Source: CAD feature listing. Evaluate the final solid. Frame: model axes, mm. Face numbers are marked on the shaded views. A direction names the side the tool comes from. Give positions to 0.01 mm unless a question says otherwise; leave off trailing zeros. Order: outer loops, then holes, each group sorted by start corner. A loop starts at its lowest first (then second) coordinate and runs counter-clockwise, first axis right, second up.
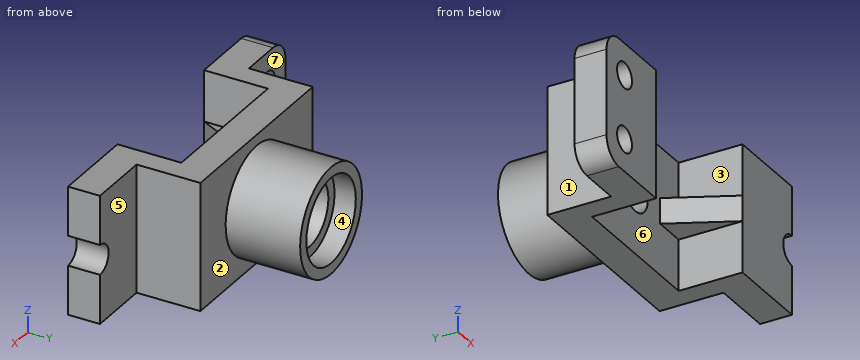
```python
from build123d import *

# Parameters (mm, degrees)
BOSS_EXTRUDE1_DEPTH = 30
BOSS_EXTRUDE2_DEPTH = 6
SKETCH3_R           = 6
CUT_EXTRUDE1_DEPTH  = 87.168439698
FILLET1_R           = 10
SKETCH4_R           = 7
CUT_EXTRUDE2_DEPTH  = 22
SKETCH5_R           = 25
BOSS_EXTRUDE3_DEPTH = 35
SKETCH6_R           = 20
CUT_EXTRUDE3_DEPTH  = 10
SKETCH7_R           = 15
SKETCH8_R           = 10


with BuildPart() as part:
    # Sketch1 → Boss-Extrude1 (new, symmetric)
    with BuildSketch(Plane.XY):
        Polygon((-75, 0), (-35, 0), (-35, 30), (35, 30), (35, 0), (75, 0), (75, 15), (45.422535211, 15), (45.422535211, 45), (-45.422535211, 45), (-45.422535211, 15), (-75, 15), align=None)
    extrude(amount=BOSS_EXTRUDE1_DEPTH, both=True)

    # Sketch2 → Boss-Extrude2 (add, symmetric)
    with BuildSketch(Plane.XY):
        Polygon((-35, 0), (-35, 30), (-20, 30), align=None)
        Polygon((20, 30), (35, 30), (35, 0), align=None)
    extrude(amount=BOSS_EXTRUDE2_DEPTH, both=True)

    # Sketch3 → Cut-Extrude1 (cut, through all)
    with BuildSketch(Plane(origin=(0, 15, 0), x_dir=(1, 0, 0), z_dir=(0, 1, 0))):
        with Locations(Location((-60.422535211, -15, 0), (0, 0, 180))):
            Circle(SKETCH3_R)
        with Locations(Location((-60.422535211, 15, 0), (0, 0, 180))):
            Circle(SKETCH3_R)
    extrude(amount=-CUT_EXTRUDE1_DEPTH, mode=Mode.SUBTRACT)

    # Fillet1
    fillet1_edges = [part.edges().sort_by_distance(p)[0] for p in [
        (-75, 7.5, -30),
        (-75, 7.5, 30),
    ]]
    fillet(fillet1_edges, radius=FILLET1_R)

    # Sketch4 → Cut-Extrude2 (cut)
    with BuildSketch(Plane(origin=(0, 15, 0), x_dir=(1, 0, 0), z_dir=(0, 1, 0))):
        with Locations((75, 0)):
            Circle(SKETCH4_R)
    extrude(amount=-CUT_EXTRUDE2_DEPTH, mode=Mode.SUBTRACT)

    # Sketch5 → Boss-Extrude3 (add)
    with BuildSketch(Plane(origin=(0, 45, 0), x_dir=(1, 0, 0), z_dir=(0, 1, 0))):
        with Locations(Location((0, 0, 0), (0, 0, 270))):
            Circle(SKETCH5_R)
    extrude(amount=BOSS_EXTRUDE3_DEPTH)

    # Sketch6 → Cut-Extrude3 (cut)
    with BuildSketch(Plane(origin=(0, 80, 0), x_dir=(1, 0, 0), z_dir=(0, 1, 0))):
        with Locations(Location((0, 0, 0), (0, 0, 270))):
            Circle(SKETCH6_R)
    extrude(amount=-CUT_EXTRUDE3_DEPTH, mode=Mode.SUBTRACT)

    # Sketch7 → Cut-Loft1 section 0
    with BuildSketch(Plane(origin=(0, 70, 0), x_dir=(1, 0, 0), z_dir=(0, 1, 0))):
        Circle(SKETCH7_R)
    # Sketch8 → Cut-Loft1 section 1
    with BuildSketch(Plane.XZ.offset(-30)):
        Circle(SKETCH8_R)
    loft(mode=Mode.SUBTRACT)


solid = part.part
```
1) Pin query (flat end, axial travel): pin 1 (9 mm diameter, centred on x = 64, z = -7, fed in from +Y); pin 2 (8 mm diameter, centred on x = 3, y = 70.5, fed in from +Z); pin 3 (7.5 mm diameter, centred on x = 31, y = 13.5, fed in from +Z). Return the tip coordinate at first contact, or that it passes through.
Report:
pin 1: stops at y = 15
pin 2: stops at z = 25
pin 3: stops at z = 6
2) Reachability of the marked faces 5, 6 and 7 from +Z, -Z, +X, -X, +Y, -Y: full face, straight path, thin tool, end or side. Return the list, or none.
Report:
face 5: +Z, -Z, +X, +Y
face 6: -Y
face 7: +Z, -Z, -X, +Y
3) Section query D-D, the plane y = 35. Return the cut outline in (x, z) (3 decimals).
Report:
outline: (-45.423, -30) - (45.423, -30) - (45.423, 30) - (-45.423, 30) - close; hole circle Ø21.25 at (0, 0)
4) Material intervals for L1, parallel to X at y = 75, z = 0; L2, parallel to X at y = 4, z = 8; L3, parallel to X at y = 37.5, z = 23.5, sorted ascending.
Report:
L1: x = -25 to -20, 20 to 25
L2: x = -75 to -35, 35 to 75
L3: x = -45.42 to 45.42
5) Draft query along X for the marked faces 1, 2, 3 and 4. Return one class per face: +X half, -X half, draft (parallel to the pull), parting line (faces both ways), or undercut.
Report:
face 1: -X half
face 2: draft
face 3: undercut
face 4: undercut
6) Section query A-A, the plane y = 5. Return the cut outline in (x, z), and give its area (3 significant figures).
Report:
outline: (-75, -20) arc R10 ccw to (-65, -30) - (-35, -30) - (-35, -6) - (-32.5, -6) - (-32.5, 6) - (-35, 6) - (-35, 30) - (-65, 30) arc R10 ccw to (-75, 20) - close; (32.5, -6) - (35, -6) - (35, -30) - (75, -30) - (75, -7) arc R7 cw to (75, 7) - (75, 30) - (35, 30) - (35, 6) - (32.5, 6) - close; hole circle Ø12 at (-60.42, -15); hole circle Ø12 at (-60.42, 15)
area: 4,510 mm2
7) Section query C-C, the plane x = -58. Return the cut outline in (y, z).
Report:
outline: (0, -30) - (15, -30) - (15, -20.49) - (0, -20.49) - close; (0, -9.51) - (15, -9.51) - (15, 9.51) - (0, 9.51) - close; (0, 20.49) - (15, 20.49) - (15, 30) - (0, 30) - close
8) Section query B-B, the plane x = 0. Return the cut outline in (y, z), and give its area (3 significant figures).
Report:
outline: (30, -30) - (45, -30) - (45, -25) - (80, -25) - (80, -20) - (70, -20) - (70, -15) - (30, -10) - close; (30, 10) - (70, 15) - (70, 20) - (80, 20) - (80, 25) - (45, 25) - (45, 30) - (30, 30) - close
area: 1,250 mm2
